The model under review builds one solid part; all positions refer to its coordinate system, in mm. Round coordinates to 2 decimals unless told otherwise and drop trailing zeros. Order: outer loops, then holes, each group sorted by start corner. A loop starts at its lowest first (then second) coordinate and runs counter-clockwise, first axis right, second up. Notation, with made-up numbers: M -15,65 L 11,65 A20 ccw 11,81 Z; hole C -20,23 d7. An arc over 180 degrees is marked long. Answer as a JSON object with one key per item and string values. Group by question number.
1. Add section C-C on z = 1.5. State the section outline as (x, y) points, and give its area (3 significant figures).
2. Add section B-B on x = 3.5. State the section outline as (y, z) points, and give its area (3 significant figures).
3. Add section D-D on y = 4.5. State the section outline as (x, z) points, and give its area (3 significant figures).
4. Mouldability with a two-part tool opening along Y and no side actions: class faces 1 (the face through (26, 3, 1)), 2 (the face through (21.099, 2.426, 1.521)), 3 (the face through (13, 0, 1)) as released by +Y, released by -Y, zero draft, split by the parting line, or undercut.
5. Add section A-A on y = 3.5. State the section outline as (x, z) points.
6. To check wall thickness, follow probe 1 along X at (y, z) = (3.5, 1.75); probe 2 along Y at (x, z) = (22.5, 1.8); probe 3 along X at (y, z) = (3.75, 2.65). State the ranges of each line that lie inside material, in increasing order. Write a range as [from, to].
7. Clearance check with a flat-ended pin moving along its axis: P1, Ø4, axis at x = 20, y = 1, coming from the -Z side. State where the tip first meets the part, or that it passes through.
Autodesk Inventor part; units mm, degrees
ref_plane "YZ Plane" through (0, 0, 0) normal (1, 0, 0) x (0, 1, 0)
ref_plane "XZ Plane" through (0, 0, 0) normal (0, 1, 0) x (-1, 0, 0)
ref_plane "XY Plane" through (0, 0, 0) normal (0, 0, 1) x (1, 0, 0)
sketch "Sketch1" plane through (0, 0, 0) normal (0, 0, 1) x (1, 0, 0)
  line L0 (0, 0) -> (26, 0)
  line L1 (26, 0) -> (26, 7)
  line L2 (26, 7) -> (0, 7)
  line L3 (0, 7) -> (0, 0)
  dimension "d0" = 26
  dimension "d1" = 7
extrude "Extrusion1" add sketch "Sketch1" along normal blind 3
sketch "Sketch2" plane through (0, 0, 3) normal (0, 0, 1) x (1, 0, 0)
  line L0 (0, 0) -> (26, 0)
  line L1 (26, 7) -> (0, 7)
  line L2 (0, 7) -> (3.5739, 7)
  line L3 (3.5739, 0) -> (0, 0)
  line L4 (0, 0) -> (0, 7)
  line L5 (3.5739, 0) -> (22.546, 0)
  line L6 (22.546, 7) -> (3.5739, 7)
  line L7 (22.546, 7) -> (26, 7)
  line L8 (26, 7) -> (26, 0)
  line L9 (26, 0) -> (22.546, 0)
  line L10 (0, 0) -> (3.4896, 0)
  line L11 (3.4896, 7) -> (0, 7)
  line L12 (0, 7) -> (0, 0)
  line L13 (3.4896, 7) -> (22.4896, 7)
  line L14 (22.4896, 0) -> (3.4896, 0)
  line L15 (22.4896, 0) -> (26, 0)
  line L16 (26, 0) -> (26, 7)
  line L17 (26, 7) -> (22.4896, 7)
  line L18 (0, 0) -> (3.5, 0)
  line L19 (3.5, 0) -> (3.5, 7)
  line L20 (3.5, 7) -> (0, 7)
  line L21 (0, 7) -> (0, 0)
  line L22 (3.5, 0) -> (22.5, 0)
  line L23 (22.5, 0) -> (22.5, 7)
  line L24 (22.5, 7) -> (3.5, 7)
  line L25 (3.5, 7) -> (3.5, 0)
  line L26 (26, 0) -> (22.5, 0)
  line L27 (22.5, 0) -> (22.5, 3.5)
  line L28 (22.5, 3.5) -> (26, 3.5)
  line L29 (26, 3.5) -> (26, 0)
  circle A0 centre (3.5, 3.5) radius 1.7782
  circle A1 centre (22.5, 3.5) radius 1.7655
  dimension "d13" = 3.5
  dimension "d14" = 19
  dimension "d15" = 3.5564
  dimension "d16" = 3.531
extrude "Extrusion2" cut sketch "Sketch2" against normal blind 4.25 contours A0 L19 | L19 A0 | A1 L23 | L23 L28 A1 | L23 A1 L28
properties part number "Transmitter clamp"
Recorded:
{
 "1": {"outline": "M 0,0 L 26,0 L 26,7 L 0,7 Z; hole C 3.5,3.5 d3.56; hole C 22.5,3.5 d3.53", "area": "162 mm²"},
 "2": {"outline": "M 0,0 L 1.72,0 L 1.72,3 L 0,3 Z; M 5.28,0 L 7,0 L 7,3 L 5.28,3 Z", "area": "10.3 mm²"},
 "3": {"outline": "M 0,0 L 2.03,0 L 2.03,3 L 0,3 Z; M 4.97,0 L 21.05,0 L 21.05,3 L 4.97,3 Z; M 23.95,0 L 26,0 L 26,3 L 23.95,3 Z", "area": "60.4 mm²"},
 "4": {"face 1": "zero draft", "face 2": "undercut", "face 3": "released by -Y"},
 "5": {"outline": "M 0,0 L 1.72,0 L 1.72,3 L 0,3 Z; M 5.28,0 L 20.73,0 L 20.73,3 L 5.28,3 Z; M 24.27,0 L 26,0 L 26,3 L 24.27,3 Z"},
 "6": {"probe 1": "x = [0, 1.72], [5.28, 20.73], [24.27, 26]", "probe 2": "y = [0, 1.73], [5.27, 7]", "probe 3": "x = [0, 1.74], [5.26, 20.75], [24.25, 26]"},
 "7": {"P1": "stops at z = 0"}
}
